Here's how the part is built. I have some questions about the finished solid (model axes, mm). A direction names the side the tool comes from. Give positions to 0.01 mm unless a question says otherwise; leave off trailing zeros. Loops run counter-clockwise (first coordinate to the right, second up) from the corner with the lowest first, then second, coordinate; pieces in that order, holes last. Notation, with made-up numbers: (-25, 50.5) -> (8, 50.5) arc R30 cw to (8, 83.5) -> close; hole circle Ø1 at (53, 88.5). An arc over 180 degrees is marked (long way). Answer in a Markdown table with one row per item. Add a question column.
Item 1: We'd pull the mould along Z, two halves only. Please class faces 5 (the face through (6, 23.812, -4)), 6 (the face through (9.798, 14.798, -2.922)), 7 (the face through (6.394, 52.952, -2.717)): released by +Z, released by -Z, zero draft, split by the parting line, or undercut.
Item 2: If we section it at D-D (z = -20): Write out the boundary of the cut face in (x, y).
Item 3: If I drill on line 1 (Y direction, x = 8, z = -11); line 2 (Y direction, x = 5, z = -2); line 3 (Z direction, x = 7.25, y = 36.5), over which ranges is the centre line in solid material (lowest first)?
Item 4: If we section it at C-C (y = 33): Write out the boundary of the cut face in (x, z).
Item 5: If we section it at B-B (x = 6.35): Give the number of separate pieces and of enclosed holes in the cut face, then the cut area to 3 significant figures.
Item 6: Which directions (+Z, -Z, +X, -X, +Y, -Y) give clear straight access to the entire face, cutting with the end or side of a thin tool? Please do faces 1 (the face through (2.54, 15, -4)), 2 (the face through (0.362, 26.959, -5.968)), 3 (the face through (3.175, 49, -3)), 4 (the face through (9.525, 49, -3)).
Item 7: For P1, Ø0.9, axis at y = 47, z = -2.5, coming from the +X side; P2, Ø3, axis at y = 21, z = -7.5, coming from the +X side; P3, Ø1.9, axis at y = 50, z = -4.5, coming from the -X side (3 decimals); P4, Ø12, axis at y = 28.5, z = -6.5, coming from the -X side, each with a flat end and sliding along its axis, tell me the tip position at first contact or that it passes through.
Item 8: If we section it at A-A (z = -26.67): Write out the boundary of the cut face in (x, y), then the cut area to 3 significant figures.
```python
from build123d import *

# Parameters (mm, degrees)
BOSS_EXTRUDE1_DEPTH = 12.7
SKETCH4_R           = 1.4605
CUT_EXTRUDE1_DEPTH  = 62.237182332
SKETCH7_W           = 3.175
SKETCH7_H           = 8.255
CUT_EXTRUDE3_DEPTH  = 63.399049722
SKETCH8_R           = 1.524
CUT_EXTRUDE4_DEPTH  = 12.7
CUT_EXTRUDE5_DEPTH  = 3.1496
CUT_EXTRUDE6_DEPTH  = 65.699146295
CUT_EXTRUDE7_DEPTH  = 3.81
FILLET2_R           = 1.27


with BuildPart() as part:
    # Sketch3 → Boss-Extrude1 (new body)
    with BuildSketch(Plane(origin=(0, 0, 0), x_dir=(0, 0, -1), z_dir=(1, 0, 0))):
        Polygon((0, 0), (31.75, 0), (31.75, 4.7625), (6.35, 4.7625), (6.35, 55.5625), (0, 55.5625), align=None)
    extrude(amount=BOSS_EXTRUDE1_DEPTH)

    # Sketch4 → Cut-Extrude1 (cut, through all)
    with BuildSketch(Plane(origin=(0, 4.7625, 0), x_dir=(1, 0, 0), z_dir=(0, 1, 0))):
        with Locations(Location((6.35, 26.67, 0), (0, 0, 270))):
            Circle(SKETCH4_R)
        with Locations(Location((6.35, 7.874, 0), (0, 0, 270))):
            Circle(SKETCH4_R)
    extrude(amount=-CUT_EXTRUDE1_DEPTH, mode=Mode.SUBTRACT)

    # Sketch7 → Cut-Extrude3 (cut, through all)
    with BuildSketch(Plane(origin=(0, 0, -6.35), x_dir=(-1, 0, 0), z_dir=(0, 0, -1))):
        with Locations((-11.1125, 51.435)):
            Rectangle(SKETCH7_W, SKETCH7_H)
        with Locations((-1.5875, 51.435)):
            Rectangle(SKETCH7_W, SKETCH7_H)
    extrude(amount=-CUT_EXTRUDE3_DEPTH, mode=Mode.SUBTRACT)

    # Sketch8 → Cut-Extrude4 (cut)
    with BuildSketch(Plane(origin=(9.525, 0, 0), x_dir=(0, 0, -1), z_dir=(1, 0, 0))):
        with Locations(Location((3.175, 51.4985, 0), (0, 0, 90))):
            Circle(SKETCH8_R)
    extrude(amount=-CUT_EXTRUDE4_DEPTH, mode=Mode.SUBTRACT)

    # Sketch9 → Cut-Extrude5 (cut)
    with BuildSketch(Plane(origin=(12.7, 0, 0), x_dir=(0, 0, -1), z_dir=(1, 0, 0))):
        with BuildLine():
            Line((0, 47.3075), (6.35, 47.3075))
            ThreePointArc((6.35, 47.3075), (3.175, 46.240638648), (0, 47.3075))
        make_face()
    cut_extrude5 = extrude(amount=-CUT_EXTRUDE5_DEPTH, mode=Mode.SUBTRACT)

    # Mirror1: Cut-Extrude5 across plane
    add(cut_extrude5.mirror(Plane(origin=(6.35, 0, 0), x_dir=(0, 0, 1), z_dir=(1, 0, 0))), mode=Mode.SUBTRACT)

    # Sketch10 → Cut-Extrude6 (cut, through all)
    with BuildSketch(Plane(origin=(9.525, 0, 0), x_dir=(0, 0, -1), z_dir=(1, 0, 0))):
        with BuildLine():
            Line((0, 53.099909067), (0, 55.639909067))
            Line((0, 55.639909067), (6.35, 55.639909067))
            Line((6.35, 55.639909067), (6.35, 53.099909067))
            ThreePointArc((6.35, 53.099909067), (3.175, 55.0545), (0, 53.099909067))
        make_face()
    extrude(amount=-CUT_EXTRUDE6_DEPTH, mode=Mode.SUBTRACT)

    # Sketch11 → Cut-Extrude7 (cut)
    with BuildSketch(Plane(origin=(0, 0, -6.35), x_dir=(-1, 0, 0), z_dir=(0, 0, -1))):
        Polygon((-6.35, 23.8125), (-10.16, 23.8125), (-10.16, 4.7625), (-2.54, 4.7625), (-2.54, 23.8125), align=None)
    extrude(amount=-CUT_EXTRUDE7_DEPTH, mode=Mode.SUBTRACT)

    # Fillet2
    fillet2_edges = [part.edges().sort_by_distance(p)[0] for p in [
        (12.7, 2.38125, -31.75),
        (10.16, 4.7625, -4.445),
        (6.35, 23.8125, -2.54),
        (2.54, 14.2875, -6.35),
        (6.35, 23.8125, -6.35),
        (10.16, 14.2875, -6.35),
        (11.43, 4.7625, -6.35),
        (6.35, 4.7625, -31.75),
        (12.7, 4.7625, -19.05),
        (12.7, 26.035, -6.35),
        (12.7, 23.65375, 0),
        (0, 23.65375, 0),
        (0, 26.035, -6.35),
        (0, 4.7625, -19.05),
        (0, 2.38125, -31.75),
        (1.27, 4.7625, -6.35),
        (2.54, 14.2875, -2.54),
        (6.35, 4.7625, -2.54),
        (2.54, 4.7625, -4.445),
        (10.16, 14.2875, -2.54),
    ]]
    fillet(fillet2_edges, radius=FILLET2_R - 0.0001)  # a hair under: the kernel refuses the full size


solid = part.part
```
Recorded:
| question | item | result |
|---|---|---|
| 1 | face 5 | zero draft |
| 1 | face 6 | released by -Z |
| 1 | face 7 | undercut |
| 2 | outline | (0, 0) -> (12.7, 0) -> (12.7, 3.49) arc R1.27 ccw to (11.43, 4.76) -> (1.27, 4.76) arc R1.27 ccw to (0, 3.49) -> close |
| 3 | line 1 | y = 0 to 4.76 |
| 3 | line 2 | y = 0 to 50.53, 52.47 to 54.85 |
| 3 | line 3 | z = -6.35 to 0 |
| 4 | outline | (0, -5.08) arc R1.27 ccw to (1.27, -6.35) -> (11.43, -6.35) arc R1.27 ccw to (12.7, -5.08) -> (12.7, -1.27) arc R1.27 ccw to (11.43, 0) -> (1.27, 0) arc R1.27 ccw to (0, -1.27) -> close |
| 5 | separate pieces | 3 |
| 5 | enclosed holes | 1 |
| 5 | area | 359 mm^2 |
| 6 | face 1 | -Z |
| 6 | face 2 | -Z, -X, +Y |
| 6 | face 3 | +Z, -Z, -X, +Y |
| 6 | face 4 | +Z, -Z, +X, +Y |
| 7 | P1 | stops at x = 9.55 |
| 7 | P2 | stops at x = 12.31 |
| 7 | P3 | stops at x = 3.175 |
| 7 | P4 | stops at x = 0 |
| 8 | outline | (0, 0) -> (4.89, 0) -> (4.89, 4.76) -> (1.27, 4.76) arc R1.27 ccw to (0, 3.49) -> close; (7.81, 0) -> (12.7, 0) -> (12.7, 3.49) arc R1.27 ccw to (11.43, 4.76) -> (7.81, 4.76) -> close |
| 8 | area | 45.9 mm^2 |
